```python
from build123d import *

# Parameters (mm, degrees)
BOSS_EXTRUDE1_DEPTH = 6.35
CUT_EXTRUDE1_REACH  = 8.35
SKETCH2_W           = 10
SKETCH2_H           = 6.35


with BuildPart() as part:
    # Sketch1 → Boss-Extrude1 (new body)
    with BuildSketch(Plane(origin=(0, 0, 0), x_dir=(1, 0, 0), z_dir=(0, 1, 0))):
        Polygon((0, 0), (19.4, 0), (19.4, 8.7), (23.4, 8.7), (23.4, -9.35), (-4, -9.35), (-4, 8.7), (0, 8.7), align=None)
    extrude(amount=BOSS_EXTRUDE1_DEPTH)

    # Sketch2 → Cut-Extrude1 (cut, up to next)
    with BuildSketch(Plane(origin=(0, 6.35, 0), x_dir=(1, 0, 0), z_dir=(0, 1, 0)), mode=Mode.PRIVATE) as cut_extrude1_sk1:
        with Locations((9.7, -6.175)):
            Rectangle(SKETCH2_W, SKETCH2_H)
    cut_extrude1_tool1 = extrude(cut_extrude1_sk1.sketch, amount=-CUT_EXTRUDE1_REACH, mode=Mode.PRIVATE) & part.part
    add(cut_extrude1_tool1.solids().sort_by_distance((9.7, 6.35, 6.175))[0], mode=Mode.SUBTRACT)


solid = part.part
```
Input: part model. Units: mm. Frame: model coordinates. A direction names the side the tool comes from. Coordinates: 2 decimals unless noted, no trailing zeros. Loops run counter-clockwise (first coordinate to the right, second up) from the corner with the lowest first, then second, coordinate; pieces in that order, holes last.
Q1. Line query: line 1 along X through (y, z) = (5, -2.75); line 2 along X through (y, z) = (3.25, 5.75); line 3 along Z through (x, y) = (1.5, 5.5). Output: solid intervals per line, ascending.
Results are:
line 1: x = -4 to 0, 19.4 to 23.4
line 2: x = -4 to 4.7, 14.7 to 23.4
line 3: z = 0 to 9.35
Q2. Contact query for a flat-ended pin moving along its axis: pin 1 (1.5 mm diameter, centred on x = 12.5, z = 7.5, fed in from +Y). Output: stop coordinate, or through.
Results are:
pin 1: passes through
Q3. Section C-C, the plane z = 6.75. Return the cut outline in (x, y).
Results are:
outline: (-4, 0) - (4.7, 0) - (4.7, 6.35) - (-4, 6.35) - close; (14.7, 0) - (23.4, 0) - (23.4, 6.35) - (14.7, 6.35) - close
Q4. Section A-A, the plane z = -5.5. Return the cut outline in (x, y).
Results are:
outline: (-4, 0) - (0, 0) - (0, 6.35) - (-4, 6.35) - close; (19.4, 0) - (23.4, 0) - (23.4, 6.35) - (19.4, 6.35) - close
Q5. Set-up query: faces 1 (the flat face through (10, 6.35, 2)), 2 (the flat face through (14.7, 3, 6)), 3 (the flat face through (0, 3, -4)). Return all of +Z, -Z, +X, -X, +Y, -Y with unobstructed straight access to the full face (end or side cutting, diameter ignored); none if empty.
Results are:
face 1: +Z, -Z, +X, -X, +Y
face 2: +Z, +Y, -Y
face 3: -Z, +Y, -Y
Q6. Section D-D, the plane x = 2.5. Return the cut outline in (y, z), and give its area (3 significant figures).
Results are:
outline: (0, 0) - (6.35, 0) - (6.35, 9.35) - (0, 9.35) - close
area: 59.4 mm2
Q7. Section B-B, the plane y = 5.5. Return the cut outline in (x, z).
Results are:
outline: (-4, -8.7) - (0, -8.7) - (0, 0) - (19.4, 0) - (19.4, -8.7) - (23.4, -8.7) - (23.4, 9.35) - (14.7, 9.35) - (14.7, 3) - (4.7, 3) - (4.7, 9.35) - (-4, 9.35) - close
Q8. Mould query, pull axis X, two halves, no side actions, for faces 4 (the flat face through (19.4, 3, -4)), 5 (the flat face through (0, 3, 9.35)), 6 (the flat face through (-4, 3, 0)). Classes: +X half, -X half, draft (parallel to the pull), parting line (faces both ways), or undercut.
Results are:
face 4: undercut
face 5: draft
face 6: -X half
